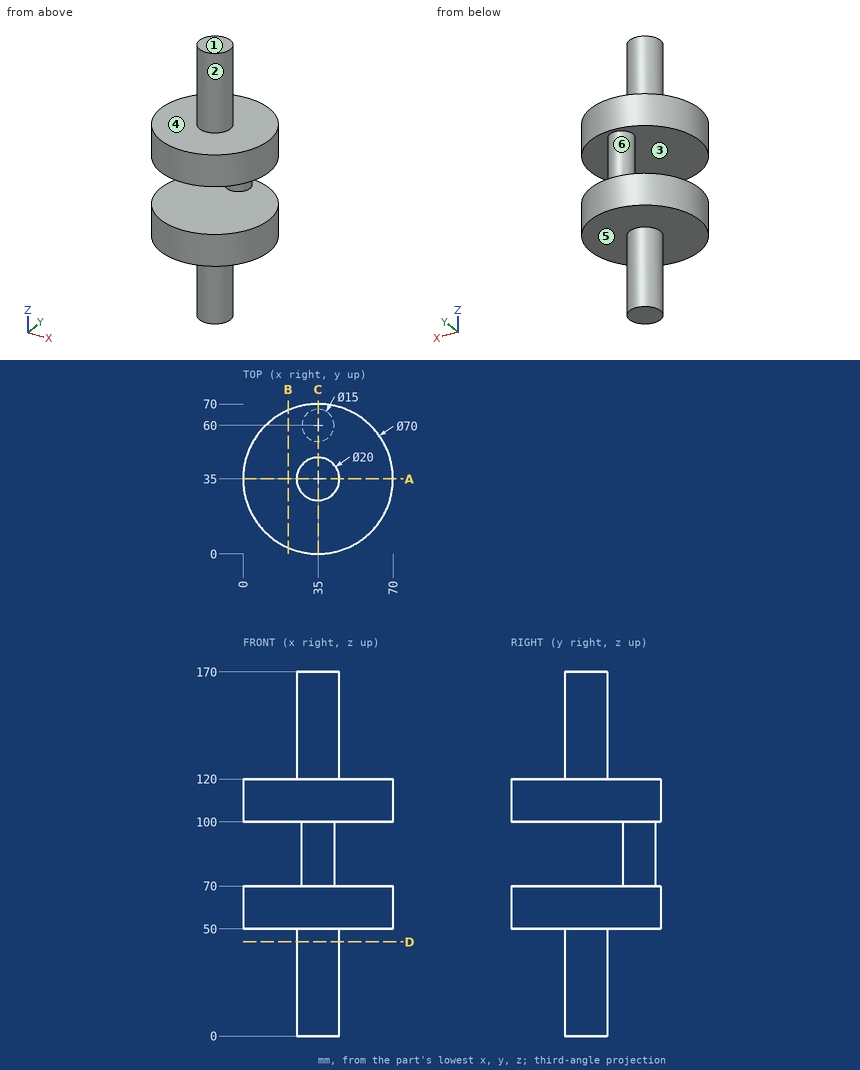
Could you check a few things on this drawing? It's one solid part, dimensions in mm from its lowest x, y, z. A direction names the side the tool comes from. Coordinates: 2 decimals unless noted, no trailing zeros. Loops run counter-clockwise (first coordinate to the right, second up) from the corner with the lowest first, then second, coordinate; pieces in that order, holes last. Notation, with made-up numbers: (38, -34) - (85, -34) arc R29 cw to (85, -10) - close; hole circle Ø2 at (-38, 84.25). An arc over 180 degrees is marked (long way). Answer as a JSON object with one key per item and string values. Group by question number.
Item 1: If we mould it in two halves opening along Z, with no side actions, what happens to the marked faces 1, 2 and 3? For each: released by +Z, released by -Z, zero draft, split by the parting line, or undercut.
Item 2: If I drill on L1, parallel to Z at x = 23.5, y = 27; L2, parallel to Y at x = 5, z = 100.5; L3, parallel to Y at x = 58.5, z = 105, over which ranges is the centre line in solid material (lowest first)? Write a range as from..to.
Item 3: For pin 1 (1 mm diameter, centred on y = 38, z = 132.5, fed in from -X); pin 2 (1.5 mm diameter, centred on x = 16.5, y = 55, fed in from -Z); pin 3 (12 mm diameter, centred on y = 13, z = 68.5, fed in from -X); pin 4 (12 mm diameter, centred on x = 44, y = 23, fed in from -Z), each with a flat end and sliding along its axis, tell me the tip position at first contact or that it passes through.
Item 4: If we section it at A-A (y = 35): List the corners of the cut face in (x, z) for me.
Item 5: If we section it at B-B (x = 21): List the corners of the cut face in (y, z) for me, plus the area to 3 significant figures.
Item 6: If we section it at D-D (z = 44): List the corners of the cut face in (x, y) for me.
Item 7: If we section it at C-C (x = 35): List the corners of the cut face in (y, z) for me, plus the area to 3 significant figures.
Item 8: On a 3-axis mill with a long thin cutter (end or side, diameter ignored), from which of +Z, -Z, +X, -X, +Y, -Y can I reach the whole of each face in a straight line? I mean the marked faces 4, 5 and 6. Say none if no direction works.
Returned:
{
 "1": {"face 1": "released by +Z", "face 2": "zero draft", "face 3": "undercut"},
 "2": {"L1": "z = 50..70, 100..120", "L2": "y = 16.97..53.03", "L3": "y = 9.06..60.94"},
 "3": {"pin 1": "stops at x = 25.32", "pin 2": "stops at z = 50", "pin 3": "stops at x = 3.87", "pin 4": "stops at z = 0"},
 "4": {"outline": "(0, 50) - (25, 50) - (25, 0) - (45, 0) - (45, 50) - (70, 50) - (70, 70) - (0, 70) - close; (0, 100) - (70, 100) - (70, 120) - (45, 120) - (45, 170) - (25, 170) - (25, 120) - (0, 120) - close"},
 "5": {"outline": "(2.92, 50) - (67.08, 50) - (67.08, 70) - (2.92, 70) - close; (2.92, 100) - (67.08, 100) - (67.08, 120) - (2.92, 120) - close", "area": "2,570 mm²"},
 "6": {"outline": "circle Ø20 at (35, 35)"},
 "7": {"outline": "(0, 50) - (25, 50) - (25, 0) - (45, 0) - (45, 50) - (70, 50) - (70, 70) - (67.5, 70) - (67.5, 100) - (70, 100) - (70, 120) - (45, 120) - (45, 170) - (25, 170) - (25, 120) - (0, 120) - (0, 100) - (52.5, 100) - (52.5, 70) - (0, 70) - close", "area": "5,250 mm²"},
 "8": {"face 4": "+Z", "face 5": "-Z", "face 6": "none"}
}
